Work out the finished part from the listing and answer in its coordinate system (mm). Give positions to 0.01 mm unless a question says otherwise; leave off trailing zeros. Loops run counter-clockwise (first coordinate to the right, second up) from the corner with the lowest first, then second, coordinate; pieces in that order, holes last. Notation, with made-up numbers: (11.5, -29) - (22.5, -29) arc R7 cw to (22.5, -23) - close; hole circle Ø8 at (78, 41.5). An arc over 180 degrees is marked (long way). Use one line per item in the form item = value. Start each with the question number.
from build123d import *

# Parameters (mm, degrees)
SKETCH1_R           = 1.5
BOSS_EXTRUDE1_DEPTH = 2


with BuildPart() as part:
    # Sketch1 → Boss-Extrude1 (new body)
    with BuildSketch(Plane(origin=(0, 0, 0), x_dir=(1, 0, 0), z_dir=(0, 1, 0))):
        with BuildLine():
            ThreePointArc((9.564996236, 77.917335601), (0.016639307, 84.999986157), (-9.555234796, 77.949150385))
            ThreePointArc((-9.555234796, 77.949150385), (-30.018823636, 52.027506279), (-62.695893908, 47.242197528))
            ThreePointArc((-62.695893908, 47.242197528), (-73.603827679, 42.514403141), (-72.283561835, 30.69949912))
            ThreePointArc((-72.283561835, 30.69949912), (-60.066553951, 0.016689279), (-72.260890144, -30.675138073))
            ThreePointArc((-72.260890144, -30.675138073), (-73.620466987, -42.485583015), (-62.728327039, -47.249651265))
            ThreePointArc((-62.728327039, -47.249651265), (-30.047730315, -52.010817), (-9.564996236, -77.917335601))
            ThreePointArc((-9.564996236, -77.917335601), (-0.016639307, -84.999986157), (9.555234796, -77.949150385))
            ThreePointArc((9.555234796, -77.949150385), (30.018823636, -52.027506279), (62.695893908, -47.242197528))
            ThreePointArc((62.695893908, -47.242197528), (73.603827679, -42.514403141), (72.283561835, -30.69949912))
            ThreePointArc((72.283561835, -30.69949912), (60.066553951, -0.016689279), (72.260890144, 30.675138073))
            ThreePointArc((72.260890144, 30.675138073), (73.620466987, 42.485583015), (62.728327039, 47.249651265))
            ThreePointArc((62.728327039, 47.249651265), (30.047730315, 52.010817), (9.564996236, 77.917335601))
        make_face()
        with Locations(Location((-64.951905284, -37.5, 0), (0, 0, 90))):
            Circle(SKETCH1_R, mode=Mode.SUBTRACT)
        with Locations(Location((0, 75, 0), (0, 0, 90))):
            Circle(SKETCH1_R, mode=Mode.SUBTRACT)
        with Locations(Location((-25, 43.301270189, 0), (0, 0, 90))):
            Circle(SKETCH1_R, mode=Mode.SUBTRACT)
        with Locations(Location((-64.951905284, 37.5, 0), (0, 0, 90))):
            Circle(SKETCH1_R, mode=Mode.SUBTRACT)
        with Locations(Location((64.951905284, 37.5, 0), (0, 0, 90))):
            Circle(SKETCH1_R, mode=Mode.SUBTRACT)
        with Locations(Location((64.951905284, -37.5, 0), (0, 0, 90))):
            Circle(SKETCH1_R, mode=Mode.SUBTRACT)
        with Locations(Location((25, 43.301270189, 0), (0, 0, 90))):
            Circle(SKETCH1_R, mode=Mode.SUBTRACT)
        with Locations(Location((0, -75, 0), (0, 0, 90))):
            Circle(SKETCH1_R, mode=Mode.SUBTRACT)
        with Locations(Location((-50, 0, 0), (0, 0, 90))):
            Circle(SKETCH1_R, mode=Mode.SUBTRACT)
        with Locations(Location((25, -43.301270189, 0), (0, 0, 90))):
            Circle(SKETCH1_R, mode=Mode.SUBTRACT)
        with Locations(Location((-25, -43.301270189, 0), (0, 0, 90))):
            Circle(SKETCH1_R, mode=Mode.SUBTRACT)
        with Locations(Location((50, 0, 0), (0, 0, 90))):
            Circle(SKETCH1_R, mode=Mode.SUBTRACT)
    extrude(amount=BOSS_EXTRUDE1_DEPTH)


solid = part.part
1) A cutting plane is placed at A-A (y = 1.05). State how many separate pieces and enclosed holes the cut face has, plus the area to 3 significant figures.
2) A cutting plane is placed at B-B (z = -19.5). Give the vertices of the cut face in (x, y).
3) A flat-ended cylindrical pin translates along its axis: pin 1 Ø5 at (x, z) = (64.95, -37.5) entering from -Y. Find the tip coordinate at first contact, or state that the pin passes through.
4) Find the intervals of material crossed by probe 1 along X at (y, z) = (1.5, 37.5); probe 2 along X at (y, z) = (1.8, -78); probe 3 along Z at (x, y) = (64.5, 0.8), in increasing order.
5) Determine the mould class of faces 1 (the flat face through (-1, 0, -1)), 2 (the cylindrical face through (30.459, 0.986, -51.776)), 3 (the cylindrical face through (73.51, 0.99, 42.67)) for opening direction Z: released by +Z, released by -Z, zero draft, split by the parting line, or undercut.
6) A cutting plane is placed at C-C (x = -12.5). Give the vertices of the cut face in (y, z), plus the area to 3 significant figures.
Answer sheet:
q1.separate_pieces = 1
q1.enclosed_holes = 12
q1.area = 15,200 mm²
q2.outline = (-64.55, 0) - (64.55, 0) - (64.55, 2) - (-64.55, 2) - close
q3.pin_1 = 0
q4.probe_1 = -74.95 to -66.45, -63.45 to 63.45, 66.45 to 74.95
q4.probe_2 = -9.54 to 9.54
q4.probe_3 = -47.49 to -38.93, -36.07 to -19.4, 19.4 to 36.07, 38.93 to 47.49
q5.face_1 = zero draft
q5.face_2 = released by -Z
q5.face_3 = undercut
q6.outline = (0, -70.55) - (2, -70.55) - (2, 70.55) - (0, 70.55) - close
q6.area = 282 mm²
